Check sheet for the modelled part. Datum: model origin and axes. Units: mm. A direction names the side the tool comes from. Give positions to 0.01 mm unless a question says otherwise; leave off trailing zeros. Loops run counter-clockwise (first coordinate to the right, second up) from the corner with the lowest first, then second, coordinate; pieces in that order, holes last. Notation, with made-up numbers: M 19,39 L 45,39 A17 cw 45,66 Z; hole C -10.5,-5 d8. An arc over 180 degrees is marked long. Put each result on its own line as item: value. Start each with the question number.
```python
from build123d import *

# Parameters (mm, degrees)
SKETCH1_W           = 254
SKETCH1_H           = 31.75
SKETCH1_R           = 7.9375
BOSS_EXTRUDE1_DEPTH = 12.7


with BuildPart() as part:
    # Sketch1 → Boss-Extrude1 (new body)
    with BuildSketch(Plane(origin=(0, 0, 0), x_dir=(1, 0, 0), z_dir=(0, 1, 0))):
        with Locations((-127, -15.875)):
            Rectangle(SKETCH1_W, SKETCH1_H)
        with Locations(Location((-19.05, -15.875, 0), (0, 0, 270))):
            Circle(SKETCH1_R, mode=Mode.SUBTRACT)
        with BuildLine():
            Line((-234.95, -9.525), (-69.85, -9.525))
            ThreePointArc((-69.85, -9.525), (-63.5, -15.875), (-69.85, -22.225))
            Line((-69.85, -22.225), (-234.95, -22.225))
            ThreePointArc((-234.95, -22.225), (-241.3, -15.875), (-234.95, -9.525))
        make_face(mode=Mode.SUBTRACT)
    extrude(amount=BOSS_EXTRUDE1_DEPTH)


solid = part.part
```
Q1. Depth check by flat-ended pin: P1, Ø4, axis at y = 6.5, z = 8, coming from the +X side. Enter the tip coordinate at first touch or a pass-through.
Q2. Section check B-B, the plane z = 14. Record the cut outline in (x, y), then the cut area to 3 significant figures.
Q3. Access from +Z, -Z, +X, -X, +Y, -Y to the whole of each face (thin tool, end or side, straight path). Record for faces 1 (the face through (-63.5, 6.26, 15.74)), 2 (the face through (-129, 6, 0)).
Q4. Thickness scan on line 1 along Z through (x, y) = (-143.5, 3) (3 decimals); line 2 along X through (y, z) = (8.5, 14); line 3 along X through (y, z) = (4, 21.5). Record the ranges inside material, lowest first. Write a range as [from, to].
Q5. Section check D-D, the plane x = -19.05. Record the cut outline in (y, z), then the cut area to 3 significant figures.
Q6. Section check A-A, the plane x = -224. Record the cut outline in (y, z) (3 decimals), then the cut area to 3 significant figures.
Q7. Section check C-C, the plane y = 9. Give the number of separate pieces and of enclosed holes in the cut face, then the cut area to 3 significant figures.
Found:
1. P1: stops at x = 0
2. outline: M -254,0 L -241.02,0 L -241.02,12.7 L -254,12.7 Z; M -63.78,0 L -26.76,0 L -26.76,12.7 L -63.78,12.7 Z; M -11.34,0 L 0,0 L 0,12.7 L -11.34,12.7 Z
2. area: 779 mm^2
3. face 1: +Y, -Y
3. face 2: -Z, +X, -X, +Y, -Y
4. line 1: z = [0, 9.525], [22.225, 31.75]
4. line 2: x = [-254, -241.02], [-63.78, -26.76], [-11.34, 0]
4. line 3: x = [-254, -237.9], [-66.9, -24.65], [-13.45, 0]
5. outline: M 0,0 L 12.7,0 L 12.7,7.94 L 0,7.94 Z; M 0,23.81 L 12.7,23.81 L 12.7,31.75 L 0,31.75 Z
5. area: 202 mm^2
6. outline: M 0,0 L 12.7,0 L 12.7,9.525 L 0,9.525 Z; M 0,22.225 L 12.7,22.225 L 12.7,31.75 L 0,31.75 Z
6. area: 242 mm^2
7. separate pieces: 1
7. enclosed holes: 2
7. area: 5,640 mm^2
